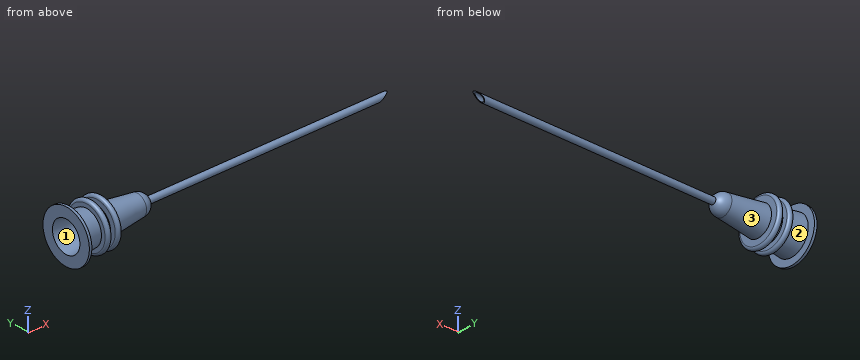
```python
from build123d import *

# Parameters (mm, degrees)
D_ME1_FACE_RADIUS       = 2
D_ME1_HEIGHT            = 2
ESQUISSE2_R             = 0.5
ENL_V_MAT_EXTRU_1_DEPTH = 10
ESQUISSE3_R             = 0.625
ESQUISSE3_R_2           = 0.5
EXTRU_MINCE1_DEPTH      = 50
ESQUISSE4_R             = 3.5
ENL_V_MAT_EXTRU_2_DEPTH = 25
ESQUISSE5_R             = 5
ENL_V_MAT_EXTRU_3_DEPTH = 25


with BuildPart() as part:
    # Esquisse1 → Révolution1 (revolve)
    with BuildSketch(Plane.XY):
        with BuildLine():
            Line((0, 0), (-1, 0))
            Line((-1, 0), (-1, 1.3674178))
            Line((-1, 1.3674178), (-14, 2.9674178))
            Line((-14, 2.9674178), (-14, 5))
            Line((-14, 5), (-13.5, 5))
            Line((-13.5, 5), (-13.5, 3.661538462))
            Line((-13.5, 3.661538462), (-10, 3.230769231))
            Line((-10, 3.230769231), (-10, 4))
            ThreePointArc((-10, 4), (-9.5, 4.5), (-9, 4))
            Line((-9, 4), (-9, 3.107692308))
            Line((-9, 3.107692308), (-8, 2.984615385))
            Line((-8, 2.984615385), (-8, 4))
            ThreePointArc((-8, 4), (-7.5, 4.5), (-7, 4))
            Line((-7, 4), (-7, 2.861538462))
            Line((-7, 2.861538462), (0, 2))
            Line((0, 2), (0, 0))
        make_face()
    revolve(axis=Axis((18.517191928, 0, 0), (-1, 0, 0)))

    # Dôme1: a dome of height H over a round flat face of radius A is a cap of a sphere of radius (A * A + H * H) / (2 * H)
    d_me1_r = (D_ME1_FACE_RADIUS * D_ME1_FACE_RADIUS + D_ME1_HEIGHT * D_ME1_HEIGHT) / (2 * D_ME1_HEIGHT)
    d_me1_base = Plane((0, 0, 0), z_dir=(1, 0, 0))
    with Locations(d_me1_base.offset(D_ME1_HEIGHT - d_me1_r)):
        d_me1_ball = Sphere(d_me1_r, mode=Mode.PRIVATE)
    add(split(d_me1_ball, bisect_by=d_me1_base, keep=Keep.TOP, mode=Mode.PRIVATE))

    # Esquisse2 → Enlèv. mat.-Extru.1 (cut)
    with BuildSketch(Plane.ZY.offset(1)):
        with Locations(Location((0, 0, 0), (0, 0, 270))):
            Circle(ESQUISSE2_R)
    extrude(amount=-ENL_V_MAT_EXTRU_1_DEPTH, mode=Mode.SUBTRACT)

    # Esquisse3 → Extru.-Mince1 (add)
    with BuildSketch(Plane.ZY.offset(1)):
        Circle(ESQUISSE3_R)
        Circle(ESQUISSE3_R_2, mode=Mode.SUBTRACT)
    extrude(amount=-EXTRU_MINCE1_DEPTH)

    # Esquisse4 → Enlèv. mat.-Extru.2 (cut, symmetric)
    with BuildSketch(Plane(origin=(0, 0, 0), x_dir=(1, 0, 0), z_dir=(0, 1, 0))):
        with Locations((49, 3.5)):
            Circle(ESQUISSE4_R)
    extrude(amount=ENL_V_MAT_EXTRU_2_DEPTH, both=True, mode=Mode.SUBTRACT)

    # Esquisse5 → Enlèv. mat.-Extru.3 (cut, symmetric)
    with BuildSketch(Plane(origin=(0, 0, 0), x_dir=(1, 0, 0), z_dir=(0, 1, 0))):
        with Locations((50.566966107, 4.123117229)):
            Circle(ESQUISSE5_R)
    extrude(amount=ENL_V_MAT_EXTRU_3_DEPTH, both=True, mode=Mode.SUBTRACT)


solid = part.part
```
Build history of the part. All positions in model axes, mm. Face numbers are marked on the shaded views. Round coordinates to 2 decimals unless told otherwise and drop trailing zeros. Loops run counter-clockwise (first coordinate to the right, second up) from the corner with the lowest first, then second, coordinate; pieces in that order, holes last.
Item 1: Saw through at B-B (x = -4.5). List the corners of the cut face in (y, z), then the cut area to 3 significant figures.
Item 2: Saw through at A-A (x = 34.5). List the corners of the cut face in (y, z) (3 decimals).
Item 3: Two-plate mould, pull along X, no slides. Class the marked faces 1, 2 and 3: released by +X, released by -X, zero draft, split by the parting line, or undercut.
Item 4: Pin check, flat tips, straight feed: P1, Ø1, axis at x = 10, y = 1.5, coming from the -Z side; P2, Ø3, axis at x = 0, z = 0.5, coming from the -Y side; P3, Ø1, axis at y = -1.5, z = 0, coming from the +X side; P4, Ø4, axis at y = 1, z = 2, coming from the +X side. Stop position of each tip, or through.
Item 5: Drill centre lines: line 1 along X through (y, z) = (-0.5, -4); line 2 along X through (y, z) = (-3.25, 2.75); line 3 along X through (y, z) = (3.25, 3.75). Where is each one in solid material? Low to high.
Worked answers:
1. outline: circle Ø5.11 at (0, 0); hole circle Ø3.6 at (0, 0)
1. area: 10.3 mm2
2. outline: circle Ø1.25 at (0, 0); hole circle Ø1 at (0, 0)
3. face 1: released by -X
3. face 2: undercut
3. face 3: released by +X
4. P1: passes through
4. P2: stops at y = -2.18
4. P3: stops at x = 1.73
4. P4: stops at x = 49
5. line 1: x = -14 to -13.5, -10 to -9, -8 to -7
5. line 2: x = -14 to -13.5, -9.93 to -9.07, -7.93 to -7.07
5. line 3: x = -14 to -13.5
